Source: CAD feature listing. Evaluate the final solid. Frame: model axes, mm. A direction names the side the tool comes from. Give positions to 0.01 mm unless a question says otherwise; leave off trailing zeros. Order: outer loops, then holes, each group sorted by start corner. A loop starts at its lowest first (then second) coordinate and runs counter-clockwise, first axis right, second up. Notation, with made-up numbers: (8.5, 62.5) - (37.5, 62.5) arc R35 cw to (37.5, 99.5) - close; hole circle Ø5 at (73, 53). An arc over 180 degrees is marked (long way). One line per item, written item: value. Start each with the question number.
from build123d import *

# Parameters (mm, degrees)
BOSS_EXTRU_1_DEPTH = 30
ESQUISSE2_R        = 2
BOSS_EXTRU_2_DEPTH = 10
BOSS_EXTRU_3_START = 10
ESQUISSE3_R        = 2
BOSS_EXTRU_3_DEPTH = 10
CHANFREIN1_SIZE    = 0.5


with BuildPart() as part:
    # Esquisse1 → Boss.-Extru.1 (new body)
    with BuildSketch(Plane.XY):
        Polygon((-3.464101615, 0), (-1.732050808, 3), (1.732050808, 3), (3.464101615, 0), (1.732050808, -3), (-1.732050808, -3), align=None)
    extrude(amount=BOSS_EXTRU_1_DEPTH)

    # Esquisse2 → Boss.-Extru.2 (add)
    with BuildSketch(Plane.XY.offset(30)):
        with Locations(Location((0, 0, 0), (0, 0, 180))):
            Circle(ESQUISSE2_R)
    extrude(amount=BOSS_EXTRU_2_DEPTH)

    # Esquisse3 → Boss.-Extru.3 (add)
    with BuildSketch(Plane(origin=(0, 0, 0), x_dir=(-1, 0, 0), z_dir=(0, 0, -1)).offset(BOSS_EXTRU_3_START)):
        Circle(ESQUISSE3_R)
    extrude(amount=-BOSS_EXTRU_3_DEPTH)

    # Chanfrein1
    chanfrein1_edges = [part.edges().sort_by_distance(p)[0] for p in [
        (2, 0, 40),
        (2, 0, -10),
    ]]
    chamfer(chanfrein1_edges, length=CHANFREIN1_SIZE)


solid = part.part
1. Contact query for a flat-ended pin moving along its axis: pin 1 Ø1.5 at (y, z) = (2.5, 10.5) entering from -X. Output: stop coordinate, or through.
2. Set-up query: faces 1 (the flat face through (-1, 2, 30)), 2 (the cylindrical face through (0, -2, -5)), 3 (the flat face through (0, 0, 40)). Return all of +Z, -Z, +X, -X, +Y, -Y with unobstructed straight access to the full face (end or side cutting, diameter ignored); none if empty.
3. Section A-A on x = 0. Return the cut outline in (y, z).
4. Section B-B on z = 24. Return the cut outline in (x, y), then the cut area to 3 significant figures.
5. Ray query, L1, parallel to Z at x = 2, y = 1; L2, parallel to Y at x = -1, z = -2.5; L3, parallel to Y at x = -2, z = 10.5. Return the intervals inside material, ascending.
6. Section C-C on z = 35.5. Return the cut outline in (x, y), then the cut area to 3 significant figures.
Data:
1. pin 1: stops at x = -2.45
2. face 1: +Z
2. face 2: -Z
2. face 3: +Z, +X, -X, +Y, -Y
3. outline: (-3, 0) - (-2, 0) - (-2, -9.5) - (-1.5, -10) - (1.5, -10) - (2, -9.5) - (2, 0) - (3, 0) - (3, 30) - (2, 30) - (2, 39.5) - (1.5, 40) - (-1.5, 40) - (-2, 39.5) - (-2, 30) - (-3, 30) - close
4. outline: (-3.46, 0) - (-1.73, -3) - (1.73, -3) - (3.46, 0) - (1.73, 3) - (-1.73, 3) - close
4. area: 31.2 mm2
5. L1: z = 0 to 30
5. L2: y = -1.73 to 1.73
5. L3: y = -2.54 to 2.54
6. outline: circle Ø4 at (0, 0)
6. area: 12.6 mm2
